CAD build for the part. Positions are in the model's coordinates, mm. Round coordinates to 2 decimals unless told otherwise and drop trailing zeros. Order: outer loops, then holes, each group sorted by start corner. A loop starts at its lowest first (then second) coordinate and runs counter-clockwise, first axis right, second up. Notation, with made-up numbers: M -5,-34 L 45,-34 A18 ccw 45,-6 Z; hole C -13.75,-35 d4. An arc over 180 degrees is marked long. Answer as CSV lines item,"result". Start each with the question number.
```python
from build123d import *

# Parameters (mm, degrees)
PAD_DEPTH              = 1.6
SKETCH001_R            = 1.75
POCKET_DEPTH           = 5
SKETCH003_W            = 6
SKETCH003_H            = 11.25
POCKET001_DEPTH        = 5
LINEARPATTERN_COUNT    = 8
LINEARPATTERN_PITCH    = 18.014286
SKETCH004_W            = 6.75
SKETCH004_H            = 7.75
POCKET002_DEPTH        = 5
LINEARPATTERN001_COUNT = 8
LINEARPATTERN001_PITCH = 18.014286


with BuildPart() as part:
    # Sketch → Pad (new body)
    with BuildSketch(Plane.XY):
        with BuildLine():
            Line((-76, 31.5), (76, 31.5))
            ThreePointArc((80, 27.5), (78.828427, 30.328427), (76, 31.5))
            Line((80, 27.5), (80, -27.5))
            ThreePointArc((76, -31.5), (78.828427, -30.328427), (80, -27.5))
            Line((76, -31.5), (-76, -31.5))
            ThreePointArc((-80, -27.5), (-78.828427, -30.328427), (-76, -31.5))
            Line((-80, -27.5), (-80, 27.5))
            ThreePointArc((-76, 31.5), (-78.828427, 30.328427), (-80, 27.5))
        make_face()
    extrude(amount=-PAD_DEPTH)

    # Sketch001 → Pocket (cut)
    with BuildSketch(Plane.XY):
        with Locations((75, 25)):
            Circle(SKETCH001_R)
        with Locations((-75, 25)):
            Circle(SKETCH001_R)
        with Locations((75, -25)):
            Circle(SKETCH001_R)
        with Locations((-75, -25)):
            Circle(SKETCH001_R)
    extrude(amount=-POCKET_DEPTH, mode=Mode.SUBTRACT)

    # Sketch003 → Pocket001 (cut)
    with BuildSketch(Plane.XY):
        with Locations((63, -19.535)):
            Rectangle(SKETCH003_W, SKETCH003_H)
    pocket001 = extrude(amount=-POCKET001_DEPTH, mode=Mode.SUBTRACT)

    # LinearPattern: Pocket001 ×8
    with Locations(*[(-i * LINEARPATTERN_PITCH, 0, 0) for i in range(1, LINEARPATTERN_COUNT)]):
        add(pocket001, mode=Mode.SUBTRACT)

    # Sketch004 → Pocket002 (cut)
    with BuildSketch(Plane.XY):
        with Locations((63, 28.765)):
            Rectangle(SKETCH004_W, SKETCH004_H)
    pocket002 = extrude(amount=-POCKET002_DEPTH, mode=Mode.SUBTRACT)

    # LinearPattern001: Pocket002 ×8
    with Locations(*[(-i * LINEARPATTERN001_PITCH, 0, 0) for i in range(1, LINEARPATTERN001_COUNT)]):
        add(pocket002, mode=Mode.SUBTRACT)


solid = part.part
```
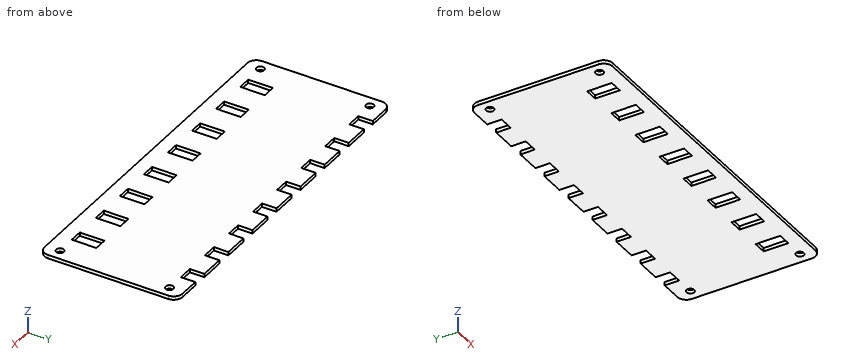
Q1. Band-saw the part on B-B, the plane y = -16. Count the separate pieces of the cut face and the enclosed holes in it, then the cut area to 3 significant figures.
Q2. Probe line 1 along Y through (x, z) = (75, -1.15); line 2 along Y through (x, z) = (-64.5, -0.3); line 3 along X through (y, z) = (24, -1). List the from-to ranges inside material, lowest first. Write a range as from..to.
Q3. Band-saw the part on A-A, the plane x = -27. Write the cut outline in (y, z).
Q4. Drop a flat-ended pin along its axis: P1, Ø0.5, axis at x = 44.5, z = -1, coming from the +Y side. Give the stop position or say it passes through.
Answer:
1,separate pieces,"9"
1,enclosed holes,"0"
1,area,"179 mm^2"
2,line 1,"y = -31.5..-26.75, -23.25..23.25, 26.75..31.5"
2,line 2,"y = -31.5..-25.16, -13.91..24.89"
2,line 3,"x = -80..-76.44, -73.56..73.56, 76.44..80"
3,outline,"M -31.5,-1.6 L -25.16,-1.6 L -25.16,0 L -31.5,0 Z; M -13.91,-1.6 L 24.89,-1.6 L 24.89,0 L -13.91,0 Z"
4,P1,"stops at y = 24.89"
